Work out the finished part from the listing and answer in its coordinate system (mm). Face numbers are marked on the shaded views. Round coordinates to 2 decimals unless told otherwise and drop trailing zeros. Order: outer loops, then holes, each group sorted by start corner. A loop starts at its lowest first (then second) coordinate and runs counter-clockwise, first axis right, second up. Notation, with made-up numbers: M 18.5,44 L 53.5,44 A32 ccw 53.5,82 Z; hole C 62,-21.75 d4. An arc over 180 degrees is marked long. Return JSON: item names as keys, results as strings.
Autodesk Inventor part; units mm, degrees
ref_plane "YZ Plane" through (0, 0, 0) normal (1, 0, 0) x (0, 1, 0)
ref_plane "XZ Plane" through (0, 0, 0) normal (0, 1, 0) x (-1, 0, 0)
ref_plane "XY Plane" through (0, 0, 0) normal (0, 0, 1) x (1, 0, 0)
sketch "Sketch1" plane through (0, 0, 0) normal (0, 1, 0) x (-1, 0, 0)
  circle A0 centre (0, 0) radius 6.5
  circle A1 centre (0, 0) radius 4
  dimension "d0" = 13
  dimension "d1" = 8
extrude "Extrusion1" add sketch "Sketch1" along normal blind 7
sketch "Sketch2" plane through (0, 7, 0) normal (0, 1, 0) x (1, 0, 0)
  circle A0 centre (0, 0) radius 4.5144
  circle A1 centre (0, 0) radius 7.9884
extrude "Extrusion2" cut sketch "Sketch2" against normal blind 1
fillet "Fillet1" radius 2 1 edges at (-4.5144, 6, 0)
properties part number "ulozak prednji" material "Acetal Resin, Black"
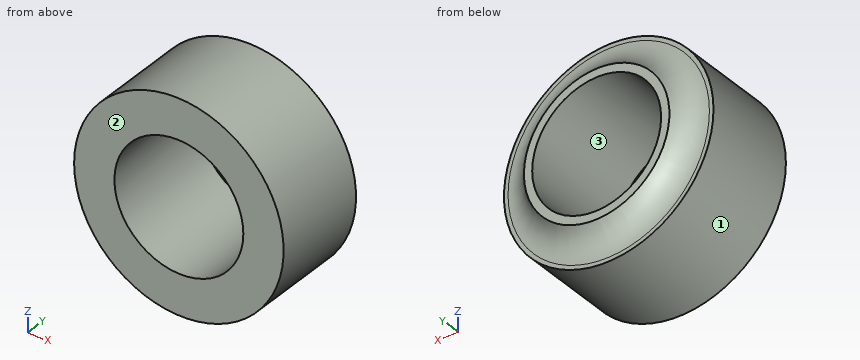
Item 1: Consider line 1 along Z through (x, y) = (0, 5.25); line 2 along X through (y, z) = (4, -0.5); line 3 along X through (y, z) = (1.25, -3). Determine where each line is inside the solid, lowest interval first. Write a range as [from, to].
Output:
{"line 1": "z = [-6.5, -4], [4, 6.5]", "line 2": "x = [-6.48, -3.97], [3.97, 6.48]", "line 3": "x = [-5.77, -2.65], [2.65, 5.77]"}
Item 2: Find section A-A (z = 0). Determine the outline of the cut face in (x, y).
Output:
{"outline": "M -6.5,0 L -4,0 L -4,7 L -4.51,7 A2 cw -6.25,6 L -6.5,6 Z; M 4,0 L 6.5,0 L 6.5,6 L 6.25,6 A2 cw 4.51,7 L 4,7 Z"}
Item 3: Find section D-D (y = 6.25). Determine the outline of the cut face in (x, z).
Output:
{"outline": "C 0,0 d10.56; hole C 0,0 d8"}
Item 4: Each of these flat-tipped pins is pushed along its axis until it touches: pin 1 (2 mm diameter, centred on x = 3.5, y = 5.5, fed in from -Z); pin 2 (3 mm diameter, centred on y = 2.5, z = -3.5, fed in from +X); pin 3 (4 mm diameter, centred on x = 1.5, z = -3, fed in from +Y); pin 4 (1 mm diameter, centred on y = 3.5, z = 3.5, fed in from +X). Where does it stop, or does it pass through?
Output:
{"pin 1": "stops at z = -6", "pin 2": "stops at x = 6.18", "pin 3": "stops at y = 7", "pin 4": "stops at x = 5.77"}
Item 5: Find section B-B (x = 0). Determine the outline of the cut face in (y, z).
Output:
{"outline": "M 0,-6.5 L 6,-6.5 L 6,-6.25 A2 cw 7,-4.51 L 7,-4 L 0,-4 Z; M 0,4 L 7,4 L 7,4.51 A2 cw 6,6.25 L 6,6.5 L 0,6.5 Z"}
Item 6: The mould has two halves that part along X. Classify the marked faces 1, 2 and 3: pulls with the +X half, pulls with the -X half, needs draft (parallel to the pull), parting line crosses it, or undercut.
Output:
{"face 1": "parting line crosses it", "face 2": "needs draft", "face 3": "undercut"}
Item 7: Find section C-C (y = 4.5). Determine the outline of the cut face in (x, z), plus the area to 3 significant figures.
Output:
{"outline": "C 0,0 d13; hole C 0,0 d8", "area": "82.5 mm^2"}
